CAD build for the part. Positions are in the model's coordinates, mm. Face numbers are marked on the shaded views. A direction names the side the tool comes from. Give positions to 0.01 mm unless a question says otherwise; leave off trailing zeros. Order: outer loops, then holes, each group sorted by start corner. A loop starts at its lowest first (then second) coordinate and runs counter-clockwise, first axis right, second up.
Item 1: Two-plate mould, pull along Z, no slides. Class the marked faces 6, 7, 8 and 9: released by +Z, released by -Z, zero draft, split by the parting line, or undercut.
Item 2: Band-saw the part on A-A on z = 54.5. Give the cut face in (x, y), plus the area to 3 significant figures.
Item 3: Flat gauge pins, fed straight in: P1, Ø2, axis at y = 7.5, z = -21, coming from the +X side; P2, Ø4.5, axis at x = 0, z = -57.5, coming from the -Y side; P3, Ø5, axis at y = 6.5, z = 59, coming from the -X side. Where does each tip first touch, or does it go through?
Item 4: Band-saw the part on C-C on x = 16.5. Give the cut face in (y, z), plus the area to 3 significant figures.
Item 5: Band-saw the part on D-D on z = -34. Give the cut face in (x, y).
Item 6: Which spindle directions (+Z, -Z, +X, -X, +Y, -Y) get a long thin tool onto all of the face, cutting with end or side? Do the marked faces 1, 2, 3, 4 and 5. Say none if no direction does.
Item 7: Wall check: L1, parallel to X at y = 11.25, z = 43.5; L2, parallel to X at y = 9, z = 44; L3, parallel to X at y = 6.25, z = -11. Give the ranges that are in metal, low to high.
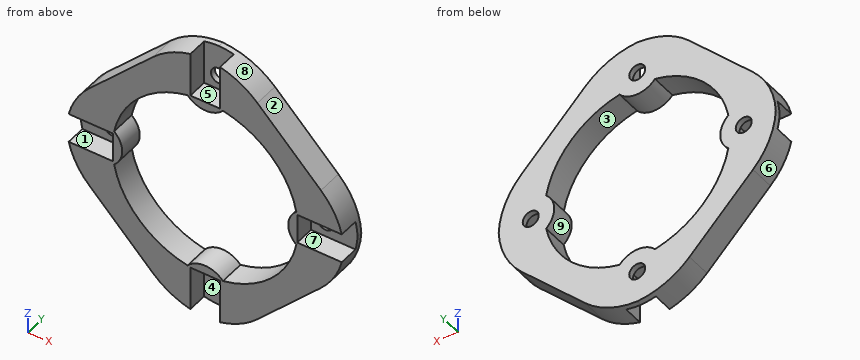
```python
from build123d import *

# Parameters (mm, degrees)
SKETCH1_R           = 72.5
SKETCH1_R_2         = 47.5
BOSS_EXTRUDE1_DEPTH = 13
SKETCH2_R           = 4.1
CUT_EXTRUDE1_DEPTH  = 104.351342517
SKETCH8_R           = 12
SKETCH8_R_2         = 4.1
BOSS_EXTRUDE4_DEPTH = 13
SKETCH3_W           = 15.2
SKETCH3_H           = 40
SKETCH3_W_2         = 40
SKETCH3_H_2         = 15.2
CUT_EXTRUDE2_DEPTH  = 10.2
BOSS_EXTRUDE2_DEPTH = 13
FILLET1_R           = 30
SKETCH7_OUTSIDE_W   = 188.094
SKETCH7_OUTSIDE_H   = 188.094
CUT_EXTRUDE4_DEPTH  = 104.351342517
FILLET3_R           = 40


with BuildPart() as part:
    # Sketch1 → Boss-Extrude1 (new body)
    with BuildSketch(Plane(origin=(0, 0, 0), x_dir=(1, 0, 0), z_dir=(0, 1, 0))):
        with Locations(Location((0, 0, 0), (0, 0, 90))):
            Circle(SKETCH1_R)
        with Locations(Location((0, 0, 0), (0, 0, 90))):
            Circle(SKETCH1_R_2, mode=Mode.SUBTRACT)
    extrude(amount=BOSS_EXTRUDE1_DEPTH)

    # Sketch2 → Cut-Extrude1 (cut, through all)
    with BuildSketch(Plane(origin=(0, 13, 0), x_dir=(1, 0, 0), z_dir=(0, 1, 0))):
        with Locations(Location((0, 54.5, 0), (0, 0, 270))):
            Circle(SKETCH2_R)
        with Locations(Location((54.5, 0, 0), (0, 0, 270))):
            Circle(SKETCH2_R)
        with Locations(Location((0, -54.5, 0), (0, 0, 270))):
            Circle(SKETCH2_R)
        with Locations(Location((-54.5, 0, 0), (0, 0, 270))):
            Circle(SKETCH2_R)
    extrude(amount=-CUT_EXTRUDE1_DEPTH, mode=Mode.SUBTRACT)

    # Sketch8 → Boss-Extrude4 (add)
    # profile 1 of 4: a face of its own
    with BuildSketch(Plane(origin=(0, 13, 0), x_dir=(1, 0, 0), z_dir=(0, 1, 0))):
        with Locations((54.5, 0)):
            Circle(SKETCH8_R)
        with Locations(Location((54.5, 0, 0), (0, 0, 270))):
            Circle(SKETCH8_R_2, mode=Mode.SUBTRACT)
    # profile 2 of 4: a face of its own
    with BuildSketch(Plane(origin=(0, 13, 0), x_dir=(1, 0, 0), z_dir=(0, 1, 0))):
        with Locations((0, -54.5)):
            Circle(SKETCH8_R)
        with Locations(Location((0, -54.5, 0), (0, 0, 270))):
            Circle(SKETCH8_R_2, mode=Mode.SUBTRACT)
    # profile 3 of 4: a face of its own
    with BuildSketch(Plane(origin=(0, 13, 0), x_dir=(1, 0, 0), z_dir=(0, 1, 0))):
        with Locations((-54.5, 0)):
            Circle(SKETCH8_R)
        with Locations(Location((-54.5, 0, 0), (0, 0, 270))):
            Circle(SKETCH8_R_2, mode=Mode.SUBTRACT)
    # profile 4 of 4: a face of its own
    with BuildSketch(Plane(origin=(0, 13, 0), x_dir=(1, 0, 0), z_dir=(0, 1, 0))):
        with Locations((0, 54.5)):
            Circle(SKETCH8_R)
        with Locations(Location((0, 54.5, 0), (0, 0, 270))):
            Circle(SKETCH8_R_2, mode=Mode.SUBTRACT)
    extrude(amount=-BOSS_EXTRUDE4_DEPTH)

    # Sketch3 → Cut-Extrude2 (cut)
    with BuildSketch(Plane.XZ):
        with Locations((0, 67.1)):
            Rectangle(SKETCH3_W, SKETCH3_H)
        with Locations((67.1, 0)):
            Rectangle(SKETCH3_W_2, SKETCH3_H_2)
        with Locations((0, -67.1)):
            Rectangle(SKETCH3_W, SKETCH3_H)
        with Locations((-67.1, 0)):
            Rectangle(SKETCH3_W_2, SKETCH3_H_2)
    extrude(amount=-CUT_EXTRUDE2_DEPTH, mode=Mode.SUBTRACT)

    # Sketch4 → Boss-Extrude2 (add)
    with BuildSketch(Plane(origin=(0, 13, 0), x_dir=(1, 0, 0), z_dir=(0, 1, 0))):
        Polygon((-38.890872965, -63.639610307), (-63.639610307, -38.890872965), (-62.123740526, -37.375003185), (-37.375003185, -62.123740526), align=None)
    extrude(amount=-BOSS_EXTRUDE2_DEPTH)

    # Fillet1
    # the kernel refuses this fillet: 30 mm, written as the material it adds along each edge
    with BuildSketch(Plane(origin=(-62.123740526, 13, 37.375003185), x_dir=(-0.46376459281913895, 0, -0.8859584654188357), z_dir=(0, -1, 0))) as fillet1_piece_1:
        with BuildLine():
            CenterArc((10.383918848, -29.947140809), FILLET1_R, 93.401739444, 18.157539937)
            Line((-0.639990933, -2.046004396), (-0.860469129, -1.487981668))
            ThreePointArc((-0.860469129, -1.487981668), (-0.892634463, -0.843880508), (-0.572638996, 0.17912169))
            Line((-0.572638996, 0.17912169), (0.035602007, 0.598942816))
            ThreePointArc((0.035602007, 0.598942816), (4.301909237, 0.472256956), (8.568216466, 0.598942816))
            Line((8.568216466, 0.598942816), (8.603818474, 0))
        make_face()
    extrude(amount=13)
    with BuildSketch(Plane(origin=(-37.375003185, 13, 62.123740526), x_dir=(0.8859584654188359, 0, 0.4637645928191383), z_dir=(0, -1, 0))) as fillet1_piece_2:
        with BuildLine():
            CenterArc((10.383918848, 29.947140809), FILLET1_R, 248.440720619, 18.157539937)
            Line((-0.639990933, 2.046004396), (-0.860469129, 1.487981668))
            ThreePointArc((-0.860469129, 1.487981668), (-0.892634463, 0.843880508), (-0.572638996, -0.17912169))
            Line((-0.572638996, -0.17912169), (0.035602007, -0.598942816))
            ThreePointArc((0.035602007, -0.598942816), (4.301909237, -0.472256956), (8.568216466, -0.598942816))
            Line((8.568216466, -0.598942816), (8.603818474, 0))
        make_face()
    extrude(amount=13)

    # Sketch7 outside → Cut-Extrude4 (cut, through all)
    with BuildSketch(Plane(origin=(0, 13, 0), x_dir=(1, 0, 0), z_dir=(0, 1, 0))):
        Rectangle(SKETCH7_OUTSIDE_W, SKETCH7_OUTSIDE_H)
        Polygon((70.931304796, -15), (15, -70.931304796), (-15, -70.931304796), (-70.931304796, -15), (-70.931304796, 15), (-15, 70.931304796), (15, 70.931304796), (70.931304796, 15), align=None, mode=Mode.SUBTRACT)
    extrude(amount=-CUT_EXTRUDE4_DEPTH, mode=Mode.SUBTRACT)

    # Fillet3
    # the kernel refuses this fillet: 40 mm, written as the material it takes off along each edge
    with BuildSketch(Plane(origin=(15, 54.421356237, 70.931304796), x_dir=(-1, 0, 0), z_dir=(0, -1, 0)), Plane(origin=(70.931304796, 54.421356237, 15), x_dir=(-0.7071067811865474, 0, 0.7071067811865476), z_dir=(0, -1, 0))) as fillet3_piece_1:
        with BuildLine():
            CenterArc((FILLET3_R * 0.414213562373, FILLET3_R), FILLET3_R, 225, 45)
            Line((-FILLET3_R * 0.292893218813, FILLET3_R * 0.292893218813), (0, 0))
            Line((0, 0), (FILLET3_R * 0.414213562373, 0))
        make_face()
    extrude(amount=95.842712475, mode=Mode.SUBTRACT)
    with BuildSketch(Plane(origin=(-15, 54.421356237, 70.931304796), x_dir=(1, 0, 0), z_dir=(0, -1, 0)), Plane(origin=(-70.931304796, 54.421356237, 15), x_dir=(0.7071067811865476, 0, 0.7071067811865476), z_dir=(0, -1, 0)), Plane(origin=(-70.931304796, 54.421356237, -15), x_dir=(0, 0, 1), z_dir=(0, -1, 0)), Plane(origin=(-15, 54.421356237, -70.931304796), x_dir=(-0.7071067811865476, 0, 0.7071067811865476), z_dir=(0, -1, 0)), Plane(origin=(15, 54.421356237, -70.931304796), x_dir=(-1, 0, 0), z_dir=(0, -1, 0)), Plane(origin=(70.931304796, 54.421356237, -15), x_dir=(-0.7071067811865476, 0, -0.7071067811865476), z_dir=(0, -1, 0))) as fillet3_piece_2:
        with BuildLine():
            CenterArc((FILLET3_R * 0.414213562373, -FILLET3_R), FILLET3_R, 90, 45)
            Line((-FILLET3_R * 0.292893218813, -FILLET3_R * 0.292893218813), (0, 0))
            Line((0, 0), (FILLET3_R * 0.414213562373, 0))
        make_face()
    extrude(amount=95.842712475, mode=Mode.SUBTRACT)


solid = part.part
```
The answers:
1. face 6: released by -Z
1. face 7: undercut
1. face 8: released by +Z
1. face 9: undercut
2. outline: (-31.43, 0) - (-7.6, 0) - (-7.6, 10.2) - (-4.1, 10.2) - (-4.1, 13) - (-31.43, 13) - close; (4.1, 10.2) - (7.6, 10.2) - (7.6, 0) - (31.43, 0) - (31.43, 13) - (4.1, 13) - close
2. area: 639 mm2
3. P1: stops at x = 64.62
3. P2: stops at y = 10.2
3. P3: stops at x = -29.43
4. outline: (0, -66.62) - (13, -66.62) - (13, -44.54) - (0, -44.54) - close; (0, 44.54) - (13, 44.54) - (13, 66.62) - (0, 66.62) - close
4. area: 574 mm2
5. outline: (-51.93, 0) - (-33.17, 0) - (-33.17, 13) - (-51.93, 13) - close; (33.17, 0) - (51.93, 0) - (51.93, 13) - (33.17, 13) - close
6. face 1: -X, -Y
6. face 2: +Z, +X, +Y, -Y
6. face 3: +Y, -Y
6. face 4: -Z, -Y
6. face 5: +Z, -Y
7. L1: x = -42.43 to -19.08, -4.8 to 4.8, 19.08 to 42.43
7. L2: x = -41.93 to -17.9, -5.81 to 5.81, 17.9 to 41.93
7. L3: x = -68.91 to -46.21, 46.21 to 68.91
